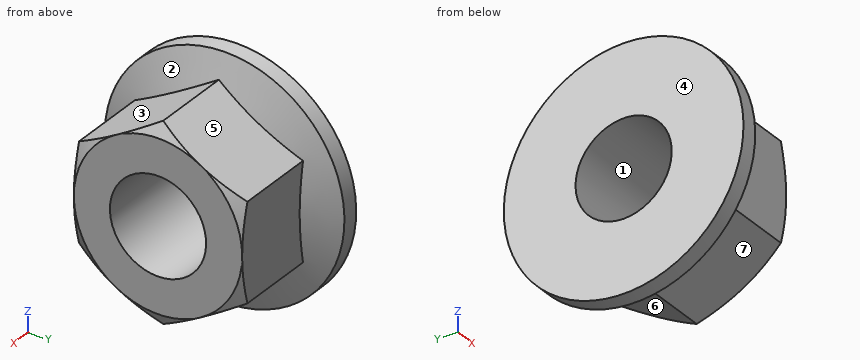
```python
from build123d import *

# Parameters (mm, degrees)
SKETCH1_R      = 6
EXTRUDE1_DEPTH = 14


# Read off the part's stored shape, not the designer's step: Cut-Extrude1
with BuildPart() as part:
    # Sketch1 → Extrude1 (new body)
    with BuildSketch(Plane(origin=(0, 0, 0), x_dir=(0, 0, -1), z_dir=(1, 0, 0))):
        Polygon((12.124355653, 0), (6.062177826, 10.5), (-6.062177826, 10.5), (-12.124355653, 0), (-6.062177826, -10.5), (6.062177826, -10.5), align=None)
        Circle(SKETCH1_R, mode=Mode.SUBTRACT)
    extrude(amount=EXTRUDE1_DEPTH)

    # Cut-Extrude1 outline → Cut-Extrude1 (revolve, cut)
    with BuildSketch(Plane.YX):
        Polygon((12.124355657, 14.000000022), (10.499999982, 14.000000022), (12.124355657, 13.062177824), align=None)
    revolve(axis=Axis((0, 0, 0), (1, 0, 0)), mode=Mode.SUBTRACT)

    # Sketch3 → Revolve1 (revolve)
    with BuildSketch(Plane.XY, mode=Mode.PRIVATE) as revolve1_sk:
        Polygon((0, 6), (0, 14.95), (2.1, 14.95), (5.357533597, 6), align=None)
    revolve(revolve1_sk.sketch.rotate(Axis((0, 0, 0), (1, 0, 0)), 90), axis=Axis((0, 0, 0), (1, 0, 0)))


solid = part.part
```
Geometry: final body of the model. Coordinates: model frame, mm. Face numbers are marked on the shaded views. A direction names the side the tool comes from. Coordinates: 2 decimals unless noted, no trailing zeros. Write each loop counter-clockwise with the first axis right and the second up, starting at its lowest first coordinate (ties: lowest second). Pieces come first, ordered by that corner, then holes. Notation, with made-up numbers: M -37.75,48 L -16.75,48 A17 cw -16.75,61 Z; hole C -28,2 d2. An arc over 180 degrees is marked long. Use CSV: the item, a comma, the result in double quotes. Start each with the question number.
1. Mould query, pull axis Z, two halves, no side actions, for the marked faces 1, 2, 3 and 4. Classes: pulls with the +Z half, pulls with the -Z half, needs draft (parallel to the pull), parting line crosses it, or undercut.
2. Reachability of the marked faces 5, 6 and 7 from +Z, -Z, +X, -X, +Y, -Y: full face, straight path, thin tool, end or side. Return the list, or none.
3. Cut plane A-A on x = 10. Return the cut outline in (y, z).
4. Ray query, probe 1 along Y at (x, z) = (4.5, 0); probe 2 along X at (y, z) = (-10.25, -6.5); probe 3 along Z at (x, y) = (1.5, 4). Return the intervals inside material, ascending.
5. First-contact query: P1, Ø5, axis at x = 7, z = 6.5, coming from the +Y side; P2, Ø1, axis at x = 11.5, z = 7, coming from the +Y side; P3, Ø2, axis at x = 12.5, y = 6, coming from the +Z side. Flat tips, straight axial feed; report the tip coordinate or a pass-through.
Entries:
1,face 1,"undercut"
1,face 2,"parting line crosses it"
1,face 3,"pulls with the +Z half"
1,face 4,"needs draft"
2,face 5,"+Z, +X, +Y"
2,face 6,"-Z, +X, +Y"
2,face 7,"-Z, +X, -Y"
3,outline,"M -10.5,-6.06 L 0,-12.12 L 10.5,-6.06 L 10.5,6.06 L 0,12.12 L -10.5,6.06 Z; hole C 0,0 d12"
4,probe 1,"-10.5 to -6, 6 to 10.5"
4,probe 2,"0 to 3.12"
4,probe 3,"-14.4 to -4.47, 4.47 to 14.4"
5,P1,"y = 10.5"
5,P2,"y = 9.74"
5,P3,"z = 9.24"
